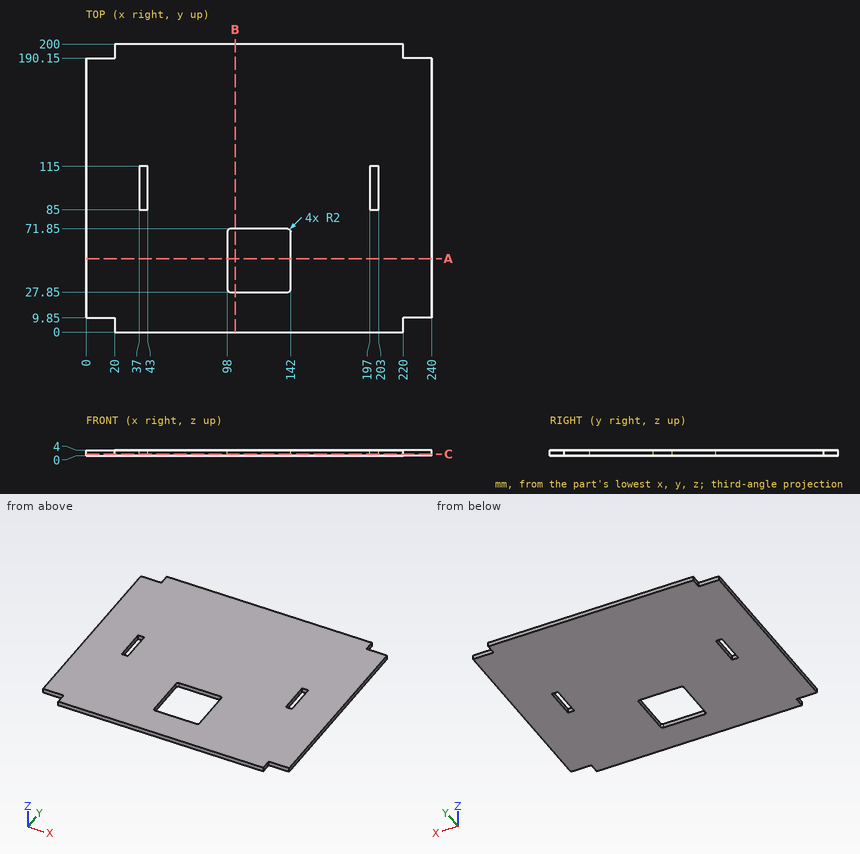
The figure shows three views and two pictorial views of one solid part (mm, origin at its lowest corner). Answer the questions. Give positions to 0.01 mm unless a question says otherwise; leave off trailing zeros. Write each loop counter-clockwise with the first axis right and the second up, starting at its lowest first coordinate (ties: lowest second). Pieces come first, ordered by that corner, then holes. Notation, with made-up numbers: (-35.75, -33) -> (13.25, -33) arc R10 cw to (13.25, -14) -> close; hole circle Ø1 at (42.5, -4). An arc over 180 degrees is marked (long way). Use one line per item in the form item = value.
1) This flat-tipped pin is pushed along its axis until it touches: P1, Ø2, axis at x = 9.5, z = 2.5, coming from the +Y side. Where does it stop, or does it pass through?
Result:
P1 = 190.15
2) Straight lines are drawn through the part: probe 1 along X at (y, z) = (111.5, 2.95); probe 2 along Y at (x, z) = (137, 0.9); probe 3 along X at (y, z) = (37.5, 0.85). For each, find the intervals that lie inside material, in ascending order.
Result:
probe_1 = 0 to 37, 43 to 197, 203 to 240
probe_2 = 0 to 27.85, 71.85 to 200
probe_3 = 0 to 98, 142 to 240
3) Section B-B on x = 103.5 is taken. Write down the section's boundary in (y, z).
Result:
outline = (0, 0) -> (27.85, 0) -> (27.85, 4) -> (0, 4) -> close; (71.85, 0) -> (200, 0) -> (200, 4) -> (71.85, 4) -> close
4) Section C-C on z = 1.35 is taken. Write down the section's boundary in (x, y).
Result:
outline = (0, 9.85) -> (20, 9.85) -> (20, 0) -> (220, 0) -> (220, 9.85) -> (240, 9.85) -> (240, 190.15) -> (220, 190.15) -> (220, 200) -> (20, 200) -> (20, 190.15) -> (0, 190.15) -> close; hole (37, 85) -> (43, 85) -> (43, 115) -> (37, 115) -> close; hole (98, 29.85) arc R2 ccw to (100, 27.85) -> (140, 27.85) arc R2 ccw to (142, 29.85) -> (142, 69.85) arc R2 ccw to (140, 71.85) -> (100, 71.85) arc R2 ccw to (98, 69.85) -> close; hole (197, 85) -> (203, 85) -> (203, 115) -> (197, 115) -> close
5) Section A-A on y = 51 is taken. Write down the section's boundary in (x, z).
Result:
outline = (0, 0) -> (98, 0) -> (98, 4) -> (0, 4) -> close; (142, 0) -> (240, 0) -> (240, 4) -> (142, 4) -> close
